```python
from build123d import *

# Parameters (mm, degrees)
SKETCH1_R           = 50.375
BOSS_EXTRUDE1_DEPTH = 9
SKETCH2_R           = 50.375
BOSS_EXTRUDE2_DEPTH = 27
SKETCH3_R           = 3
CUT_EXTRUDE3_DEPTH  = 5
SKETCH4_R           = 16
CUT_EXTRUDE4_DEPTH  = 77.185833657


with BuildPart() as part:
    # Sketch1 → Boss-Extrude1 (new body)
    with BuildSketch(Plane.XY):
        Circle(SKETCH1_R)
    extrude(amount=BOSS_EXTRUDE1_DEPTH)

    # Sketch2 → Boss-Extrude2 (add)
    with BuildSketch(Plane.XY.offset(9)):
        Circle(SKETCH2_R)
        with BuildLine():
            ThreePointArc((43.864306317, 9.470388393), (44.621611193, 4.762083526), (44.875, 0))
            ThreePointArc((44.875, 0), (44.874942611, -0.071767888), (44.874770445, -0.143535592))
            ThreePointArc((44.874770445, -0.143535592), (45.919292349, -2.043419548), (46.280875815, -4.181138531))
            ThreePointArc((46.280875815, -4.181138531), (45.662212981, -6.948786113), (43.923991772, -9.189590403))
            ThreePointArc((43.923991772, -9.189590403), (42.678661169, -13.867137623), (40.936761518, -18.383339778))
            ThreePointArc((40.936761518, -18.383339778), (41.089750325, -19.185243866), (41.141016151, -20))
            ThreePointArc((41.141016151, -20), (39.818405701, -23.929966596), (36.388820013, -26.260605535))
            ThreePointArc((36.388820013, -26.260605535), (33.348624043, -30.02723596), (29.920414626, -33.444497509))
            ThreePointArc((29.920414626, -33.444497509), (27.332014232, -37.619290238), (22.561690692, -38.790923399))
            ThreePointArc((22.561690692, -38.790923399), (18.252306858, -40.995352412), (13.730556226, -42.722797787))
            ThreePointArc((13.730556226, -42.722797787), (9.667893623, -45.483863434), (4.833440083, -44.613938203))
            ThreePointArc((4.833440083, -44.613938203), (0, -44.875), (-4.833440083, -44.613938203))
            ThreePointArc((-4.833440083, -44.613938203), (-9.667893623, -45.483863434), (-13.730556226, -42.722797787))
            ThreePointArc((-13.730556226, -42.722797787), (-18.252306858, -40.995352412), (-22.561690692, -38.790923399))
            ThreePointArc((-22.561690692, -38.790923399), (-27.332014232, -37.619290238), (-29.920414626, -33.444497509))
            ThreePointArc((-29.920414626, -33.444497509), (-33.348624043, -30.02723596), (-36.388820013, -26.260605535))
            ThreePointArc((-36.388820013, -26.260605535), (-40.270181276, -23.25), (-40.936761518, -18.383339778))
            ThreePointArc((-40.936761518, -18.383339778), (-42.678661169, -13.867137623), (-43.923991772, -9.189590403))
            ThreePointArc((-43.923991772, -9.189590403), (-46.245268135, -4.860573542), (-44.874770445, -0.143535592))
            ThreePointArc((-44.874770445, -0.143535592), (-44.629170055, 4.690714789), (-43.864306317, 9.470388393))
            ThreePointArc((-43.864306317, 9.470388393), (-44.224128008, 14.369290238), (-41.053523888, 18.121087202))
            ThreePointArc((-41.053523888, 18.121087202), (-38.862889995, 22.4375), (-36.220083805, 26.492851001))
            ThreePointArc((-36.220083805, 26.492851001), (-34.556234385, 31.114573196), (-30.133750091, 33.252409393))
            ThreePointArc((-30.133750091, 33.252409393), (-26.376863197, 36.304637623), (-22.313079754, 38.934458991))
            ThreePointArc((-22.313079754, 38.934458991), (-18.913253903, 42.47986378), (-14.003577146, 42.634087912))
            ThreePointArc((-14.003577146, 42.634087912), (-9.330037125, 43.894373583), (-4.547941505, 44.643945313))
            ThreePointArc((-4.547941505, 44.643945313), (0, 46.5), (4.547941505, 44.643945313))
            ThreePointArc((4.547941505, 44.643945313), (9.330037125, 43.894373583), (14.003577146, 42.634087912))
            ThreePointArc((14.003577146, 42.634087912), (18.913253903, 42.47986378), (22.313079754, 38.934458991))
            ThreePointArc((22.313079754, 38.934458991), (26.376863197, 36.304637623), (30.133750091, 33.252409393))
            ThreePointArc((30.133750091, 33.252409393), (34.464026918, 31.214846656), (36.225793019, 26.765224254))
            ThreePointArc((36.225793019, 26.765224254), (36.224365559, 26.629007713), (36.220083805, 26.492851001))
            ThreePointArc((36.220083805, 26.492851001), (38.862889995, 22.4375), (41.053523888, 18.121087202))
            ThreePointArc((41.053523888, 18.121087202), (43.602081289, 15.72793303), (44.542260652, 12.360679775))
            ThreePointArc((44.542260652, 12.360679775), (44.370502778, 10.876310688), (43.864306317, 9.470388393))
        make_face(mode=Mode.SUBTRACT)
    extrude(amount=BOSS_EXTRUDE2_DEPTH)

    # Sketch3 → Cut-Extrude3 (cut)
    with BuildSketch(Plane.XY.offset(9)):
        with Locations((0, 40)):
            Circle(SKETCH3_R)
        with Locations((16.269465723, 36.541818306)):
            Circle(SKETCH3_R)
        with Locations((29.725793019, 26.765224254)):
            Circle(SKETCH3_R)
        with Locations((38.042260652, 12.360679775)):
            Circle(SKETCH3_R)
        with Locations((39.780875815, -4.181138531)):
            Circle(SKETCH3_R)
        with Locations((34.641016151, -20)):
            Circle(SKETCH3_R)
        with Locations((23.511410092, -32.360679775)):
            Circle(SKETCH3_R)
        with Locations((8.316467633, -39.125904029)):
            Circle(SKETCH3_R)
        with Locations((-8.316467633, -39.125904029)):
            Circle(SKETCH3_R)
        with Locations((-23.511410092, -32.360679775)):
            Circle(SKETCH3_R)
        with Locations((-34.641016151, -20)):
            Circle(SKETCH3_R)
        with Locations((-39.780875815, -4.181138531)):
            Circle(SKETCH3_R)
        with Locations((-38.042260652, 12.360679775)):
            Circle(SKETCH3_R)
        with Locations((-29.725793019, 26.765224254)):
            Circle(SKETCH3_R)
        with Locations((-16.269465723, 36.541818306)):
            Circle(SKETCH3_R)
    extrude(amount=-CUT_EXTRUDE3_DEPTH, mode=Mode.SUBTRACT)

    # Sketch4 → Cut-Extrude4 (cut, through all)
    with BuildSketch(Plane.XY.offset(9)):
        Circle(SKETCH4_R)
    extrude(amount=-CUT_EXTRUDE4_DEPTH, mode=Mode.SUBTRACT)


solid = part.part
```
Verification items for the finished model (mm, model axes). A direction names the side the tool comes from. Give positions to 0.01 mm unless a question says otherwise; leave off trailing zeros. Write each loop counter-clockwise with the first axis right and the second up, starting at its lowest first coordinate (ties: lowest second). Pieces come first, ordered by that corner, then holes. Notation, with made-up numbers: (80.5, 81.25) - (118.5, 81.25) arc R9 cw to (118.5, 90.25) - close; hole circle Ø8 at (31, 58). An arc over 180 degrees is marked (long way). Put each result on its own line as item: value.
Q1. Scan lines: probe 1 along Y at (x, z) = (0, 5) (3 decimals); probe 2 along Y at (x, z) = (-35, 17.5); probe 3 along Y at (x, z) = (14.5, 3.5). Record each from-to range of solid material in increasing order. Write a range as from..to.
Result:
probe 1: -50.375..-16, 16..37, 43..50.375
probe 2: -36.23..-28.08, 30.56..36.23
probe 3: -48.24..-6.76, 6.76..48.24
Q2. Section check B-B on z = 7.5. Count the separate pieces of the cut face and the enclosed holes in it, and give its area (3 significant figures).
Result:
separate pieces: 1
enclosed holes: 16
area: 6,740 mm2
Q3. Section check C-C on y = 3.5. Record the cut outline in (x, z).
Result:
outline: (-50.25, 0) - (-15.61, 0) - (-15.61, 9) - (-44.74, 9) - (-44.74, 36) - (-50.25, 36) - close; (15.61, 0) - (50.25, 0) - (50.25, 36) - (44.74, 36) - (44.74, 9) - (15.61, 9) - close
Q4. Section check D-D on x = -28.5. Record the cut outline in (y, z), and give its area (3 significant figures).
Result:
outline: (-41.54, 0) - (41.54, 0) - (41.54, 36) - (34.66, 36) - (34.66, 9) - (29.5, 9) - (29.5, 4) - (24.03, 4) - (24.03, 9) - (-36.53, 9) - (-36.53, 36) - (-41.54, 36) - close
area: 1,040 mm2
Q5. Section check A-A on x = 0. Record the cut outline in (y, z) (3 decimals).
Result:
outline: (-50.375, 0) - (-16, 0) - (-16, 9) - (-44.875, 9) - (-44.875, 36) - (-50.375, 36) - close; (16, 0) - (50.375, 0) - (50.375, 36) - (46.5, 36) - (46.5, 9) - (43, 9) - (43, 4) - (37, 4) - (37, 9) - (16, 9) - close
Q6. Mould release check, pull along Y, two halves, no side actions. Record for faces 1 (the face through (18.849, 42.508, 22.311)), 2 (the face through (-6.558, 49.946, 17.748)): released by +Y, released by -Y, zero draft, split by the parting line, or undercut.
Result:
face 1: undercut
face 2: split by the parting line
Q7. Depth check by flat-ended pin: P1, Ø3, axis at x = -29.5, y = 25.5, coming from the +Z side; P2, Ø12, axis at x = -16.5, y = -37.5, coming from the +Z side; P3, Ø9.5, axis at x = 39.78, y = -4.18, coming from the +Z side; P4, Ø5, axis at y = 26.5, z = 29, coming from the -X side. Enter the tip coordinate at first touch or a pass-through.
Result:
P1: z = 4
P2: z = 36
P3: z = 9
P4: x = -44.29
Q8. Set-up check for faces 3 (the face through (-3.47, -15.62, 4.56)), 4 (the face through (38.829, 22.496, 22.311)): record each of +Z, -Z, +X, -X, +Y, -Y from which the full face is reachable in a straight line by a thin tool's end or side.
Result:
face 3: +Z, -Z
face 4: +Z
